Job drawing, mm, ordinate dimensions from the low corner. One solid piece. A direction names the side the tool comes from. Give positions to 0.01 mm unless a question says otherwise; leave off trailing zeros. Order: outer loops, then holes, each group sorted by start corner. A loop starts at its lowest first (then second) coordinate and runs counter-clockwise, first axis right, second up. Notation, with made-up numbers: M 13.5,23.5 L 68.5,23.5 A12 cw 68.5,46.5 Z; hole C 60.5,-0.75 d5. An arc over 180 degrees is marked long. Put each result on its own line as item: value. Start each with the question number.
1) Tool access for the marked faces 1 and 2: list every direction of +Z, -Z, +X, -X, +Y, -Y with a clear straight run to the whole face (end or side of a thin tool).
2) Pin check, flat tip, straight feed: pin 1 (5.5 mm diameter, centred on x = 7, y = 7, fed in from +Z). Stop position of the tip, or through.
3) Cut at C-C (z = 0.9). Write the cut outline in (x, y), and give its area (3 significant figures).
4) Drill centre lines: line 1 (Y direction, x = 7, z = 1.15); line 2 (Y direction, x = 7, z = 0.2); line 3 (Z direction, x = 7.5, y = 1.25). Where is each one in solid material? Low to high. Write a range as [from, to].
5) Cut at A-A (x = 7). Write the cut outline in (y, z), and give its area (3 significant figures).
6) Cut at D-D (x = 11.25). Write the cut outline in (y, z).
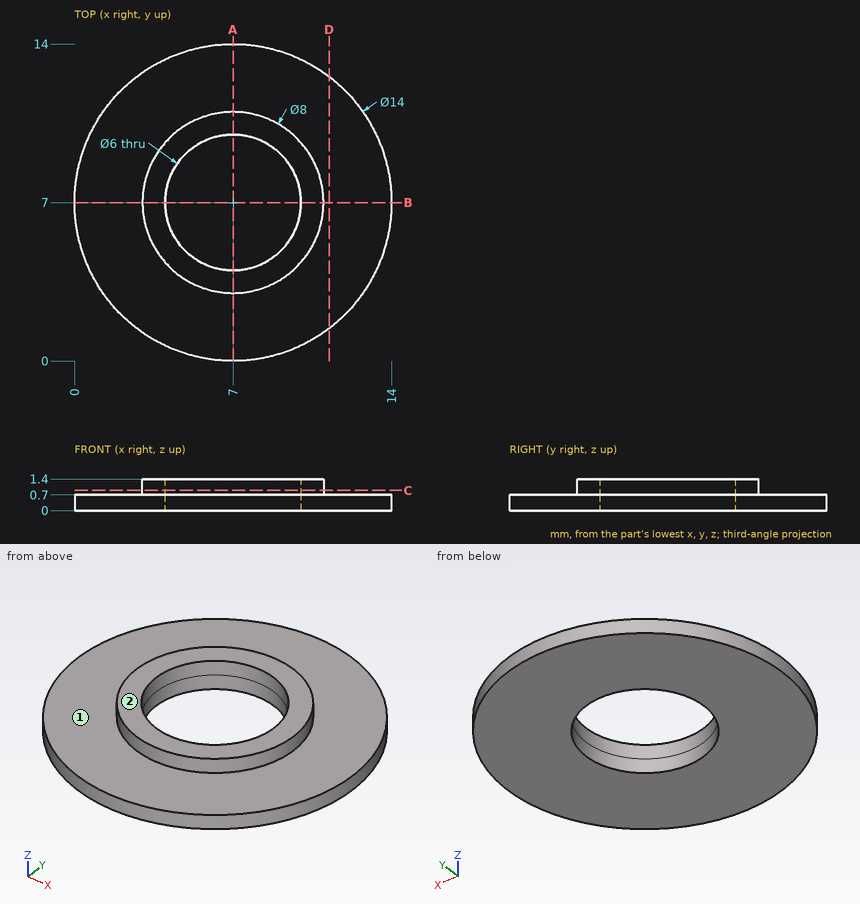
Solution:
1. face 1: +Z
1. face 2: +Z, +X, -X, +Y, -Y
2. pin 1: through
3. outline: C 7,7 d8; hole C 7,7 d6
3. area: 22.0 mm²
4. line 1: [3, 4], [10, 11]
4. line 2: [0, 4], [10, 14]
4. line 3: [0, 0.7]
5. outline: M 0,0 L 4,0 L 4,1.4 L 3,1.4 L 3,0.7 L 0,0.7 Z; M 10,0 L 14,0 L 14,0.7 L 11,0.7 L 11,1.4 L 10,1.4 Z
5. area: 7.00 mm²
6. outline: M 1.44,0 L 12.56,0 L 12.56,0.7 L 1.44,0.7 Z
